Geometry check sheet. Reference: the model listing, model coordinates, mm. Face numbers are marked on the shaded views. Round coordinates to 2 decimals unless told otherwise and drop trailing zeros. Loops run counter-clockwise (first coordinate to the right, second up) from the corner with the lowest first, then second, coordinate; pieces in that order, holes last. Notation, with made-up numbers: M 51,54 L 76,54 A15 ccw 76,64 Z; hole C 45.5,-38 d9. An arc over 180 degrees is marked long. Use one line per item in the form item = value. Start each with the question number.
1. Material ranges on line 1 (X direction, y = 8.25, z = -223.5); line 2 (Y direction, x = -166.5, z = -428), recorded low to high.
2. Cross-section at B-B (z = -352). Record the boundary of the cut face in (x, y).
3. Go/stop test with a flat-tipped pin: pin 1 (12 mm diameter, centred on x = 164, z = 17.5, fed in from +Y). Record where the tip stops, or that it passes through.
4. Draft check along X on the marked faces 1 and 2. Enter one of: pulls with the +X half, pulls with the -X half, needs draft (parallel to the pull), parting line crosses it, or undercut.
5. Cross-section at C-C (x = 133.5). Record the boundary of the cut face in (y, z).
6. Cross-section at A-A (y = 4.75). Record the boundary of the cut face in (x, z).
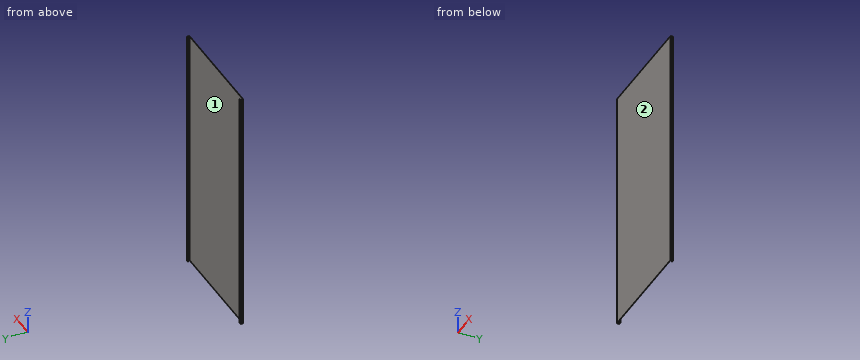
Autodesk Inventor part; units mm, degrees
ref_plane "YZ Plane" through (0, 0, 0) normal (1, 0, 0) x (0, 1, 0)
ref_plane "XZ Plane" through (0, 0, 0) normal (0, 1, 0) x (-1, 0, 0)
ref_plane "XY Plane" through (0, 0, 0) normal (0, 0, 1) x (1, 0, 0)
sketch "Sketch6" plane through (0, 0, 0) normal (0, 1, 0) x (-1, 0, 0)
  line L0 (205.5, -490) -> (-205.5, -490)
  line L1 (-205.5, -490) -> (-205.5, 490)
  line L2 (-205.5, 490) -> (205.5, 490)
  line L3 (205.5, 490) -> (205.5, -490)
  line L4 (205.5, -490) -> (-205.5, 490) construction
  line L5 (-205.5, -490) -> (205.5, 490) construction
  point P0 (0, 0)
  dimension "d52" = 411
  dimension "d53" = 980
extrude "Plate2" add sketch "Sketch6" along normal blind 0.5
sketch "Sketch11" plane through (-205, 0, 490) normal (-1, 0, 0) x (0, -1, 0)
  line L0 (0, -980) -> (0, 0)
  line L1 (0, 0) -> (-10, 0)
  line L2 (-10, 0) -> (-10, -980)
  line L3 (-10, -980) -> (0, -980)
edge flange "Flange2" height 10 angle 90 thickness 0.5 bend radius 0.5 thickness toward (-1, 0, 0) relief tear relief width 0.5 relief depth 0.25 edges at (-205.5, 0.5, 0) wall of the first edge with corners at (-205, 0, -490) (-205, 0, 490) (-205, 10, 490) (-205, 10, -490)
bend "Bend3"
corner "Corner3"
sketch "Sketch12" plane through (-205.5, 9.5, 490) normal (0, 1, 0) x (-1, 0, 0)
  line L0 (0, -980) -> (0, 0)
  line L1 (0, 0) -> (-10, 0)
  line L2 (-10, 0) -> (-10, -980)
  line L3 (-10, -980) -> (0, -980)
edge flange "Flange3" height 10 angle 90 thickness 0.5 bend radius 0.5 thickness toward (0, 1, 0) relief tear relief width 0.5 relief depth 0.25 edges at (-205, 10, 0) wall of the first edge with corners at (-205.5, 9.5, -490) (-205.5, 9.5, 490) (-195.5, 9.5, 490) (-195.5, 9.5, -490)
bend "Bend4"
corner "Corner4"
sketch "Sketch13" plane through (205, 0, -490) normal (1, 0, 0) x (0, 1, 0)
  line L0 (0, 980) -> (0, 0)
  line L1 (0, 0) -> (10, 0)
  line L2 (10, 0) -> (10, 980)
  line L3 (10, 980) -> (0, 980)
edge flange "Flange4" height 10 angle 90 thickness 0.5 bend radius 0.5 thickness toward (1, 0, 0) relief tear relief width 0.5 relief depth 0.25 edges at (205.5, 0.5, 0) wall of the first edge with corners at (205, 0, 490) (205, 0, -490) (205, 10, -490) (205, 10, 490)
bend "Bend5"
corner "Corner5"
sketch "Sketch14" plane through (205.5, 9.5, -490) normal (0, 1, 0) x (-1, 0, 0)
  line L0 (0, 980) -> (0, 0)
  line L1 (0, 0) -> (10, 0)
  line L2 (10, 0) -> (10, 980)
  line L3 (10, 980) -> (0, 980)
edge flange "Flange5" height 10 angle 90 thickness 0.5 bend radius 0.5 thickness toward (0, 1, 0) relief tear relief width 0.5 relief depth 0.25 edges at (205, 10, 0) wall of the first edge with corners at (205.5, 9.5, 490) (205.5, 9.5, -490) (195.5, 9.5, -490) (195.5, 9.5, 490)
bend "Bend6"
corner "Corner6"
fillet "Corner Round1" radius 4 4 edges at (195.5, 9.75, -490) (-195.5, 9.75, -490) (-195.5, 9.75, 490) (195.5, 9.75, 490)
equation "\"d52\" = ЖАБРЫ_базовая_ширина - 5 * ЖАБРЫ_шаг_листов"
equation "\"d53\" = ЖАБРЫ_базовая_длина_кор_лист"
equation "\"d54\" = Thickness"
equation "\"d84\" = BendReliefWidth"
equation "\"d85\" = BendReliefDepth"
equation "\"d86\" = MinimumRemnant"
equation "\"d87\" = TransitionRadius"
equation "\"d90\" = BendRadius"
equation "\"d91\" = CornerReliefSize"
equation "\"d92\" = GapSize"
equation "\"d93\" = JacobiRadiusSize"
equation "\"d94\" = BendReliefWidth"
equation "\"d95\" = BendReliefDepth"
equation "\"d96\" = MinimumRemnant"
equation "\"d97\" = TransitionRadius"
equation "\"d100\" = BendRadius"
equation "\"d101\" = CornerReliefSize"
equation "\"d102\" = GapSize"
equation "\"d103\" = JacobiRadiusSize"
equation "\"d104\" = BendReliefWidth"
equation "\"d105\" = BendReliefDepth"
equation "\"d106\" = MinimumRemnant"
equation "\"d107\" = TransitionRadius"
equation "\"d110\" = BendRadius"
equation "\"d111\" = CornerReliefSize"
equation "\"d112\" = GapSize"
equation "\"d113\" = JacobiRadiusSize"
equation "\"d114\" = BendReliefWidth"
equation "\"d115\" = BendReliefDepth"
equation "\"d116\" = MinimumRemnant"
equation "\"d117\" = TransitionRadius"
equation "\"d120\" = BendRadius"
equation "\"d121\" = CornerReliefSize"
equation "\"d122\" = GapSize"
equation "\"d123\" = JacobiRadiusSize"
equation "\"BendRadius\" = Thickness"
equation "\"BendReliefWidth\" = Thickness"
equation "\"BendReliefDepth\" = 0.5 * Thickness"
equation "\"CornerReliefSize\" = 4 * Thickness"
equation "\"MinimumRemnant\" = 2 * Thickness"
equation "\"TransitionRadius\" = BendRadius"
equation "\"JacobiRadiusSize\" = BendRadius"
equation "\"GapSize\" = Thickness"
properties part number "MSC 811 sheet gills" material "Stainless Steel"
Reported:
q1.line_1 = -205.5 to -205, 205 to 205.5
q1.line_2 = 0 to 0.5
q2.outline = M -205.5,1 A1 ccw -204.5,0 L 204.5,0 A1 ccw 205.5,1 L 205.5,9 A1 ccw 204.5,10 L 195.5,10 L 195.5,9.5 L 204.5,9.5 A0.5 cw 205,9 L 205,1 A0.5 cw 204.5,0.5 L -204.5,0.5 A0.5 cw -205,1 L -205,9 A0.5 cw -204.5,9.5 L -195.5,9.5 L -195.5,10 L -204.5,10 A1 ccw -205.5,9 Z
q3.pin_1 = 0.5
q4.face_1 = undercut
q4.face_2 = needs draft
q5.outline = M 0,-490 L 0.5,-490 L 0.5,490 L 0,490 Z
q6.outline = M -205.5,-490 L -205,-490 L -205,490 L -205.5,490 Z; M 205,-490 L 205.5,-490 L 205.5,490 L 205,490 Z
